```python
from build123d import *

# Parameters (mm, degrees)
SKETCH1_W           = 145
SKETCH1_H           = 25
BOSS_EXTRUDE1_DEPTH = 10
SKETCH2_W           = 17.5
SKETCH2_H           = 35
BOSS_EXTRUDE2_DEPTH = 10
SKETCH4_W           = 80
SKETCH4_H           = 35
BOSS_EXTRUDE3_DEPTH = 12.5
SKETCH8_R           = 2.25
CUT_EXTRUDE5_DEPTH  = 200.468042553
SKETCH9_W           = 7.3
SKETCH9_H           = 4
CUT_EXTRUDE6_DEPTH  = 10
CUT_EXTRUDE7_REACH  = 202.966
SKETCH10_R          = 3
SKETCH10_R_2        = 1.65
CHAMFER1_SIZE       = 3
FILLET1_R           = 15
SKETCH14_R          = 11.25
CUT_EXTRUDE11_DEPTH = 2.5
SKETCH15_R          = 3
CUT_EXTRUDE12_DEPTH = 2.5
CUT_EXTRUDE13_REACH = 203.835
SKETCH16_R          = 2.25
CUT_EXTRUDE15_DEPTH = 4
CUT_EXTRUDE16_REACH = 202.966
SKETCH19_W          = 60
SKETCH19_H          = 5.2
SKETCH20_R          = 1.75
CUT_EXTRUDE17_DEPTH = 202.835328919
SKETCH21_W          = 24
SKETCH21_H          = 24
CUT_EXTRUDE18_DEPTH = 2
CUT_EXTRUDE19_REACH = 203.622
SKETCH22_R          = 1.65
SKETCH22_W          = 16
SKETCH22_H          = 9
SKETCH23_R          = 3.25
CUT_EXTRUDE20_DEPTH = 3
CUT_EXTRUDE21_START = -3
SKETCH24_R          = 3.25
CUT_EXTRUDE21_DEPTH = 3


with BuildPart() as part:
    # Sketch1 → Boss-Extrude1 (new body)
    with BuildSketch(Plane(origin=(0, 0, 0), x_dir=(1, 0, 0), z_dir=(0, 1, 0))):
        with Locations((72.5, 12.5)):
            Rectangle(SKETCH1_W, SKETCH1_H)
    extrude(amount=BOSS_EXTRUDE1_DEPTH)

    # Sketch2 → Boss-Extrude2 (add)
    with BuildSketch(Plane(origin=(0, 10, 0), x_dir=(1, 0, 0), z_dir=(0, 1, 0))):
        with Locations((153.75, 17.5)):
            Rectangle(SKETCH2_W, SKETCH2_H)
    extrude(amount=-BOSS_EXTRUDE2_DEPTH)

    # Sketch4 → Boss-Extrude3 (add)
    with BuildSketch(Plane.XZ):
        with Locations((157.5, -17.5)):
            Rectangle(SKETCH4_W, SKETCH4_H)
    extrude(amount=BOSS_EXTRUDE3_DEPTH)

    # Sketch8 → Cut-Extrude5 (cut, through all)
    with BuildSketch(Plane(origin=(0, 0, -25), x_dir=(-1, 0, 0), z_dir=(0, 0, -1))):
        with Locations((-137, 5)):
            Circle(SKETCH8_R)
        with Locations((-101, 5)):
            Circle(SKETCH8_R)
        with Locations(Location((-44, 5, 0), (0, 0, 180))):
            Circle(SKETCH8_R)
        with Locations(Location((-8, 5, 0), (0, 0, 180))):
            Circle(SKETCH8_R)
    extrude(amount=-CUT_EXTRUDE5_DEPTH, mode=Mode.SUBTRACT)

    # Sketch9 → Cut-Extrude6 (cut)
    with BuildSketch(Plane(origin=(0, 10, 0), x_dir=(1, 0, 0), z_dir=(0, 1, 0))):
        with Locations((137, 20)):
            Rectangle(SKETCH9_W, SKETCH9_H)
        with Locations((137, 5)):
            Rectangle(SKETCH9_W, SKETCH9_H)
        with Locations((101, 5)):
            Rectangle(SKETCH9_W, SKETCH9_H)
        with Locations((101, 20)):
            Rectangle(SKETCH9_W, SKETCH9_H)
        with Locations((8, 20)):
            Rectangle(SKETCH9_W, SKETCH9_H)
        with Locations((44, 20)):
            Rectangle(SKETCH9_W, SKETCH9_H)
        with Locations((44, 5)):
            Rectangle(SKETCH9_W, SKETCH9_H)
        with Locations((8, 5)):
            Rectangle(SKETCH9_W, SKETCH9_H)
    extrude(amount=-CUT_EXTRUDE6_DEPTH, mode=Mode.SUBTRACT)

    # Sketch10 → Cut-Extrude7 (cut, up to next)
    with BuildSketch(Plane(origin=(0, 0, 0), x_dir=(1, 0, 0), z_dir=(0, 1, 0)), mode=Mode.PRIVATE) as cut_extrude7_sk1:
        with Locations(Location((180, 17.5, 0), (0, 0, 270))):
            Circle(SKETCH10_R)
    cut_extrude7_tool1 = extrude(cut_extrude7_sk1.sketch, amount=-CUT_EXTRUDE7_REACH, mode=Mode.PRIVATE) & part.part
    # Sketch10 → Cut-Extrude7 (cut, up to next)
    with BuildSketch(Plane(origin=(0, 0, 0), x_dir=(1, 0, 0), z_dir=(0, 1, 0)), mode=Mode.PRIVATE) as cut_extrude7_sk2:
        with Locations(Location((193, 4.5, 0), (0, 0, 270))):
            Circle(SKETCH10_R_2)
    cut_extrude7_tool2 = extrude(cut_extrude7_sk2.sketch, amount=-CUT_EXTRUDE7_REACH, mode=Mode.PRIVATE) & part.part
    # Sketch10 → Cut-Extrude7 (cut, up to next)
    with BuildSketch(Plane(origin=(0, 0, 0), x_dir=(1, 0, 0), z_dir=(0, 1, 0)), mode=Mode.PRIVATE) as cut_extrude7_sk3:
        with Locations(Location((167, 4.5, 0), (0, 0, 90))):
            Circle(SKETCH10_R_2)
    cut_extrude7_tool3 = extrude(cut_extrude7_sk3.sketch, amount=-CUT_EXTRUDE7_REACH, mode=Mode.PRIVATE) & part.part
    # Sketch10 → Cut-Extrude7 (cut, up to next)
    with BuildSketch(Plane(origin=(0, 0, 0), x_dir=(1, 0, 0), z_dir=(0, 1, 0)), mode=Mode.PRIVATE) as cut_extrude7_sk4:
        with Locations(Location((167, 30.5, 0), (0, 0, 270))):
            Circle(SKETCH10_R_2)
    cut_extrude7_tool4 = extrude(cut_extrude7_sk4.sketch, amount=-CUT_EXTRUDE7_REACH, mode=Mode.PRIVATE) & part.part
    # Sketch10 → Cut-Extrude7 (cut, up to next)
    with BuildSketch(Plane(origin=(0, 0, 0), x_dir=(1, 0, 0), z_dir=(0, 1, 0)), mode=Mode.PRIVATE) as cut_extrude7_sk5:
        with Locations(Location((193, 30.5, 0), (0, 0, 90))):
            Circle(SKETCH10_R_2)
    cut_extrude7_tool5 = extrude(cut_extrude7_sk5.sketch, amount=-CUT_EXTRUDE7_REACH, mode=Mode.PRIVATE) & part.part
    add(cut_extrude7_tool1.solids().sort_by_distance((180, 0, -17.5))[0], mode=Mode.SUBTRACT)
    add(cut_extrude7_tool2.solids().sort_by_distance((193, 0, -4.5))[0], mode=Mode.SUBTRACT)
    add(cut_extrude7_tool3.solids().sort_by_distance((167, 0, -4.5))[0], mode=Mode.SUBTRACT)
    add(cut_extrude7_tool4.solids().sort_by_distance((167, 0, -30.5))[0], mode=Mode.SUBTRACT)
    add(cut_extrude7_tool5.solids().sort_by_distance((193, 0, -30.5))[0], mode=Mode.SUBTRACT)

    # Chamfer1
    chamfer1_edges = [part.edges().sort_by_distance(p)[0] for p in [
        (197.5, -6.25, -35),
        (197.5, -6.25, 0),
    ]]
    chamfer(chamfer1_edges, length=CHAMFER1_SIZE)

    # Fillet1
    fillet1_edges = [part.edges().sort_by_distance(p)[0] for p in [
        (162.5, 5, -35),
        (162.5, 5, 0),
    ]]
    fillet(fillet1_edges, radius=FILLET1_R)

    # Sketch14 → Cut-Extrude11 (cut)
    with BuildSketch(Plane.XZ.offset(12.5)):
        with Locations(Location((180, -17.5, 0), (0, 0, 270))):
            Circle(SKETCH14_R)
    extrude(amount=-CUT_EXTRUDE11_DEPTH, mode=Mode.SUBTRACT)

    # Sketch15 → Cut-Extrude12 (cut)
    with BuildSketch(Plane(origin=(0, 0, 0), x_dir=(1, 0, 0), z_dir=(0, 1, 0))):
        with Locations(Location((167, 30.5, 0), (0, 0, 270))):
            Circle(SKETCH15_R)
        with Locations(Location((193, 30.5, 0), (0, 0, 90))):
            Circle(SKETCH15_R)
        with Locations(Location((193, 4.5, 0), (0, 0, 270))):
            Circle(SKETCH15_R)
        with Locations(Location((167, 4.5, 0), (0, 0, 90))):
            Circle(SKETCH15_R)
    extrude(amount=-CUT_EXTRUDE12_DEPTH, mode=Mode.SUBTRACT)

    # Sketch16 → Cut-Extrude13 (cut, up to next)
    with BuildSketch(Plane(origin=(0, 10, 0), x_dir=(1, 0, 0), z_dir=(0, 1, 0)), mode=Mode.PRIVATE) as cut_extrude13_sk1:
        with Locations(Location((57.5, 12.5, 0), (0, 0, 270))):
            Circle(SKETCH16_R)
    cut_extrude13_tool1 = extrude(cut_extrude13_sk1.sketch, amount=-CUT_EXTRUDE13_REACH, mode=Mode.PRIVATE) & part.part
    # Sketch16 → Cut-Extrude13 (cut, up to next)
    with BuildSketch(Plane(origin=(0, 10, 0), x_dir=(1, 0, 0), z_dir=(0, 1, 0)), mode=Mode.PRIVATE) as cut_extrude13_sk2:
        with Locations(Location((87.5, 12.5, 0), (0, 0, 270))):
            Circle(SKETCH16_R)
    cut_extrude13_tool2 = extrude(cut_extrude13_sk2.sketch, amount=-CUT_EXTRUDE13_REACH, mode=Mode.PRIVATE) & part.part
    add(cut_extrude13_tool1.solids().sort_by_distance((57.5, 10, -12.5))[0], mode=Mode.SUBTRACT)
    add(cut_extrude13_tool2.solids().sort_by_distance((87.5, 10, -12.5))[0], mode=Mode.SUBTRACT)

    # Sketch18 → Cut-Extrude15 (cut)
    with BuildSketch(Plane(origin=(0, 10, 0), x_dir=(1, 0, 0), z_dir=(0, 1, 0))):
        Polygon((83.285343035, 12.5), (85.392671517, 8.85), (89.607328483, 8.85), (91.714656965, 12.5), (89.607328483, 16.15), (85.392671517, 16.15), align=None)
        Polygon((59.607328483, 16.15), (61.714656965, 12.5), (59.607328483, 8.85), (55.392671517, 8.85), (53.285343035, 12.5), (55.392671517, 16.15), align=None)
    extrude(amount=-CUT_EXTRUDE15_DEPTH, mode=Mode.SUBTRACT)

    # Sketch19 → Cut-Extrude16 (cut, up to next)
    with BuildSketch(Plane.XY, mode=Mode.PRIVATE) as cut_extrude16_sk1:
        with Locations((164.5, -6.25)):
            Rectangle(SKETCH19_W, SKETCH19_H)
    cut_extrude16_tool1 = extrude(cut_extrude16_sk1.sketch, amount=-CUT_EXTRUDE16_REACH, mode=Mode.PRIVATE) & part.part
    add(cut_extrude16_tool1.solids().sort_by_distance((164.5, -6.25, 0))[0], mode=Mode.SUBTRACT)

    # Sketch20 → Cut-Extrude17 (cut, through all)
    with BuildSketch(Plane(origin=(0, 10, 0), x_dir=(1, 0, 0), z_dir=(0, 1, 0))):
        with Locations(Location((152, 17.5, 0), (0, 0, 270))):
            Circle(SKETCH20_R)
    extrude(amount=-CUT_EXTRUDE17_DEPTH, mode=Mode.SUBTRACT)

    # Sketch21 → Cut-Extrude18 (cut)
    with BuildSketch(Plane.XZ.offset(12.5)):
        with Locations((152, -17.5)):
            Rectangle(SKETCH21_W, SKETCH21_H)
    extrude(amount=-CUT_EXTRUDE18_DEPTH, mode=Mode.SUBTRACT)

    # Sketch22 → Cut-Extrude19 (cut, up to next)
    with BuildSketch(Plane.XZ.offset(10.5), mode=Mode.PRIVATE) as cut_extrude19_sk1:
        with Locations(Location((144, -9.5, 0), (0, 0, 270))):
            Circle(SKETCH22_R)
    cut_extrude19_tool1 = extrude(cut_extrude19_sk1.sketch, amount=-CUT_EXTRUDE19_REACH, mode=Mode.PRIVATE) & part.part
    # Sketch22 → Cut-Extrude19 (cut, up to next)
    with BuildSketch(Plane.XZ.offset(10.5), mode=Mode.PRIVATE) as cut_extrude19_sk2:
        with Locations(Location((160, -9.5, 0), (0, 0, 270))):
            Circle(SKETCH22_R)
    cut_extrude19_tool2 = extrude(cut_extrude19_sk2.sketch, amount=-CUT_EXTRUDE19_REACH, mode=Mode.PRIVATE) & part.part
    # Sketch22 → Cut-Extrude19 (cut, up to next)
    with BuildSketch(Plane.XZ.offset(10.5), mode=Mode.PRIVATE) as cut_extrude19_sk3:
        with Locations(Location((160, -25.5, 0), (0, 0, 270))):
            Circle(SKETCH22_R)
    cut_extrude19_tool3 = extrude(cut_extrude19_sk3.sketch, amount=-CUT_EXTRUDE19_REACH, mode=Mode.PRIVATE) & part.part
    # Sketch22 → Cut-Extrude19 (cut, up to next)
    with BuildSketch(Plane.XZ.offset(10.5), mode=Mode.PRIVATE) as cut_extrude19_sk4:
        with Locations(Location((144, -25.5, 0), (0, 0, 270))):
            Circle(SKETCH22_R)
    cut_extrude19_tool4 = extrude(cut_extrude19_sk4.sketch, amount=-CUT_EXTRUDE19_REACH, mode=Mode.PRIVATE) & part.part
    # Sketch22 → Cut-Extrude19 (cut, up to next)
    with BuildSketch(Plane.XZ.offset(10.5), mode=Mode.PRIVATE) as cut_extrude19_sk5:
        with Locations((152, -17.5)):
            Rectangle(SKETCH22_W, SKETCH22_H)
    cut_extrude19_tool5 = extrude(cut_extrude19_sk5.sketch, amount=-CUT_EXTRUDE19_REACH, mode=Mode.PRIVATE) & part.part
    add(cut_extrude19_tool1.solids().sort_by_distance((144, -10.5, -9.5))[0], mode=Mode.SUBTRACT)
    add(cut_extrude19_tool2.solids().sort_by_distance((160, -10.5, -9.5))[0], mode=Mode.SUBTRACT)
    add(cut_extrude19_tool3.solids().sort_by_distance((160, -10.5, -25.5))[0], mode=Mode.SUBTRACT)
    add(cut_extrude19_tool4.solids().sort_by_distance((144, -10.5, -25.5))[0], mode=Mode.SUBTRACT)
    add(cut_extrude19_tool5.solids().sort_by_distance((152, -10.5, -17.5))[0], mode=Mode.SUBTRACT)

    # Sketch23 → Cut-Extrude20 (cut)
    with BuildSketch(Plane(origin=(0, 10, 0), x_dir=(1, 0, 0), z_dir=(0, 1, 0))):
        with Locations(Location((152, 17.5, 0), (0, 0, 270))):
            Circle(SKETCH23_R)
    extrude(amount=-CUT_EXTRUDE20_DEPTH, mode=Mode.SUBTRACT)

    # Sketch24 → Cut-Extrude21 (cut)
    with BuildSketch(Plane.XZ.offset(3.65).offset(CUT_EXTRUDE21_START)):
        with Locations(Location((152, -17.5, 0), (0, 0, 90))):
            Circle(SKETCH24_R)
    extrude(amount=CUT_EXTRUDE21_DEPTH, mode=Mode.SUBTRACT)


solid = part.part
```
Read the model definition and answer for the solid it produces. Units are mm, in the model's axes. A direction names the side the tool comes from. Coordinates: 2 decimals unless noted, no trailing zeros. Write each loop counter-clockwise with the first axis right and the second up, starting at its lowest first coordinate (ties: lowest second). Pieces come first, ordered by that corner, then holes. Notation, with made-up numbers: (2, -13) - (15, -13) arc R26 cw to (15, 19) - close; hole circle Ø10 at (45.25, 28). An arc over 180 degrees is marked (long way). Answer as a JSON object with one key per item and string values. Group by question number.
1. The mould has two halves that part along X. Classify faces 5 (the flat face through (7.1, 7.3, -3)), 6 (the flat face through (96, 1, 0)): +X half, -X half, draft (parallel to the pull), parting line (faces both ways), or undercut.
2. Each of these flat-tipped pins is pushed along its axis until it touches: P1, Ø3.5, axis at x = 10, y = 5, coming from the -Z side; P2, Ø2, axis at x = 37, z = -19.5, coming from the -Y side; P3, Ø1.2, axis at x = 135.5, z = -19.5, coming from the +Y side. Where does it stop, or does it pass through?
3. Consider L1, parallel to X at y = -2.6, z = -17.5; L2, parallel to X at y = -11, z = -17.5; L3, parallel to Z at x = 167, y = -10.7. Determine where each line is inside the solid, lowest interval first. Write a range as [from, to].
4. A cutting plane is placed at B-B (x = 137). Give the number of separate pieces and of enclosed holes in the cut face, plus the area to 3 significant figures.
5. A cutting plane is placed at A-A (x = 8). Determine the outline of the cut face in (y, z).
6. Which of the six approach directions +Z, -Z, +X, -X, +Y, -Y give full straight-line access (tool end or side, diameter ignored) to faces 1 (the cylindrical face through (154.197, 8.521, -19.895)), 2 (the flat face through (43.1, 7.3, -22)), 3 (the flat face through (134.5, -6, -17)), 4 (the flat face through (178, -10, -20))?
7. A cutting plane is placed at D-D (x = 33). Determine the outline of the cut face in (y, z).
Worked out:
{
 "1": {"face 5": "undercut", "face 6": "draft"},
 "2": {"P1": "stops at z = -25", "P2": "stops at y = 0", "P3": "stops at y = 0"},
 "3": {"L1": "x = [117.5, 148.75], [155.25, 177], [183, 197.5]", "L2": "x = [117.5, 140], [164, 168.75], [191.25, 197.5]", "L3": "z = [-35, -32.15], [-28.85, -6.15], [-2.85, 0]"},
 "4": {"separate pieces": "5", "enclosed holes": "0", "area": "349 mm²"},
 "5": {"outline": "(0, -25) - (2.75, -25) - (2.75, -22) - (0, -22) - close; (0, -18) - (2.75, -18) - (2.75, -7) - (0, -7) - close; (0, -3) - (2.75, -3) - (2.75, 0) - (0, 0) - close; (7.25, -25) - (10, -25) - (10, -22) - (7.25, -22) - close; (7.25, -18) - (10, -18) - (10, -7) - (7.25, -7) - close; (7.25, -3) - (10, -3) - (10, 0) - (7.25, 0) - close"},
 "6": {"face 1": "+Y", "face 2": "+Y, -Y", "face 3": "+Z, -Z", "face 4": "-Y"},
 "7": {"outline": "(0, -25) - (10, -25) - (10, 0) - (0, 0) - close"}
}
